Read the model definition and answer for the solid it produces. Units are mm, in the model's axes. Face numbers are marked on the shaded views. A direction names the side the tool comes from. Coordinates: 2 decimals unless noted, no trailing zeros. Order: outer loops, then holes, each group sorted by start corner. A loop starts at its lowest first (then second) coordinate and runs counter-clockwise, first axis right, second up.
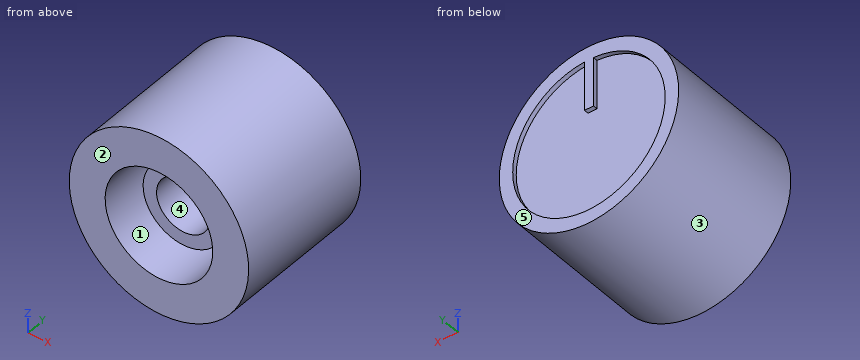
from build123d import *

# Parameters (mm, degrees)
SKETCH_2_W      = 1
SKETCH_2_H      = 5.5
EXTRUDE_1_DEPTH = 0.5


with BuildPart() as part:
    # Эскиз1 → Повернуть1 (revolve)
    with BuildSketch(Plane(origin=(0, 0, 0), x_dir=(0, 0, -1), z_dir=(1, 0, 0))):
        Polygon((0, 0), (-3, 0), (-3, -9.5), (-4.5, -9.5), (-4.5, -2), (-6, -2), (-6, -13), (-10, -13), (-10, 3), (-8.5, 3), (-8.5, 2.5), (0, 2.5), align=None)
    revolve(axis=Axis((0, 2.5, 0), (0, -1, 0)))

    # Эскиз2 → Бобышка-Вытянуть1 (add)
    with BuildSketch(Plane(origin=(0, 2.5, 0), x_dir=(1, 0, 0), z_dir=(0, 1, 0))):
        with Locations((0, -5.75)):
            Rectangle(SKETCH_2_W, SKETCH_2_H)
    extrude(amount=EXTRUDE_1_DEPTH)


solid = part.part
Q1. The part is cut by section D-D, the plane y = -0.5. Determine the outline of the cut face in (x, z).
Q2. The part is cut by section B-B, the plane y = -8.25. Determine the outline of the cut face in (x, z), then the cut area to 3 significant figures.
Q3. The part is cut by section A-A, the plane x = 0. Determine the outline of the cut face in (y, z).
Q4. Each of these flat-tipped pins is pushed along its axis until it touches: P1, Ø7, axis at x = 0, z = 0, coming from the +Y side; P2, Ø3, axis at y = -10.5, z = -2.5, coming from the +X side; P3, Ø3.5, axis at x = -3, z = -1.5, coming from the -Y side; P4, Ø1.5, axis at y = -8, z = -3.5, coming from the +X side. Where does it stop, or does it pass through?
Q5. Determine the mould class of the marked faces 3, 4 and 5 for opening direction Z: +Z half, -Z half, draft (parallel to the pull), parting line (faces both ways), or undercut.
Q6. The part is cut by section C-C, the plane z = 0. Determine the outline of the cut face in (x, y).
Q7. Which of the six approach directions +Z, -Z, +X, -X, +Y, -Y give full straight-line access (tool end or side, diameter ignored) to the marked faces 1 and 2?
Q8. Straight lines are drawn through the part: L1, parallel to X at y = -6.5, z = 0; L2, parallel to Z at x = 0, y = -10.25. For each, find the intervals that lie inside material, in ascending order.
Computed values:
1. outline: circle Ø20 at (0, 0); hole circle Ø6 at (0, 0)
2. outline: circle Ø20 at (0, 0); circle Ø9 at (0, 0); hole circle Ø12 at (0, 0); hole circle Ø6 at (0, 0)
2. area: 236 mm2
3. outline: (-13, -10) - (3, -10) - (3, -8.5) - (2.5, -8.5) - (2.5, 3) - (3, 3) - (3, 10) - (-13, 10) - (-13, 6) - (-2, 6) - (-2, 4.5) - (-9.5, 4.5) - (-9.5, 3) - (0, 3) - (0, -3) - (-9.5, -3) - (-9.5, -4.5) - (-2, -4.5) - (-2, -6) - (-13, -6) - close
4. P1: stops at y = 3
4. P2: stops at x = 9.95
4. P3: stops at y = -9.5
4. P4: stops at x = 9.61
5. face 3: parting line
5. face 4: undercut
5. face 5: draft
6. outline: (-10, -13) - (-6, -13) - (-6, -2) - (-4.5, -2) - (-4.5, -9.5) - (-3, -9.5) - (-3, 0) - (3, 0) - (3, -9.5) - (4.5, -9.5) - (4.5, -2) - (6, -2) - (6, -13) - (10, -13) - (10, 3) - (8.5, 3) - (8.5, 2.5) - (-8.5, 2.5) - (-8.5, 3) - (-10, 3) - close
7. face 1: -Y
7. face 2: +Z, -Z, +X, -X, -Y
8. L1: x = -10 to -6, -4.5 to -3, 3 to 4.5, 6 to 10
8. L2: z = -10 to -6, 6 to 10
